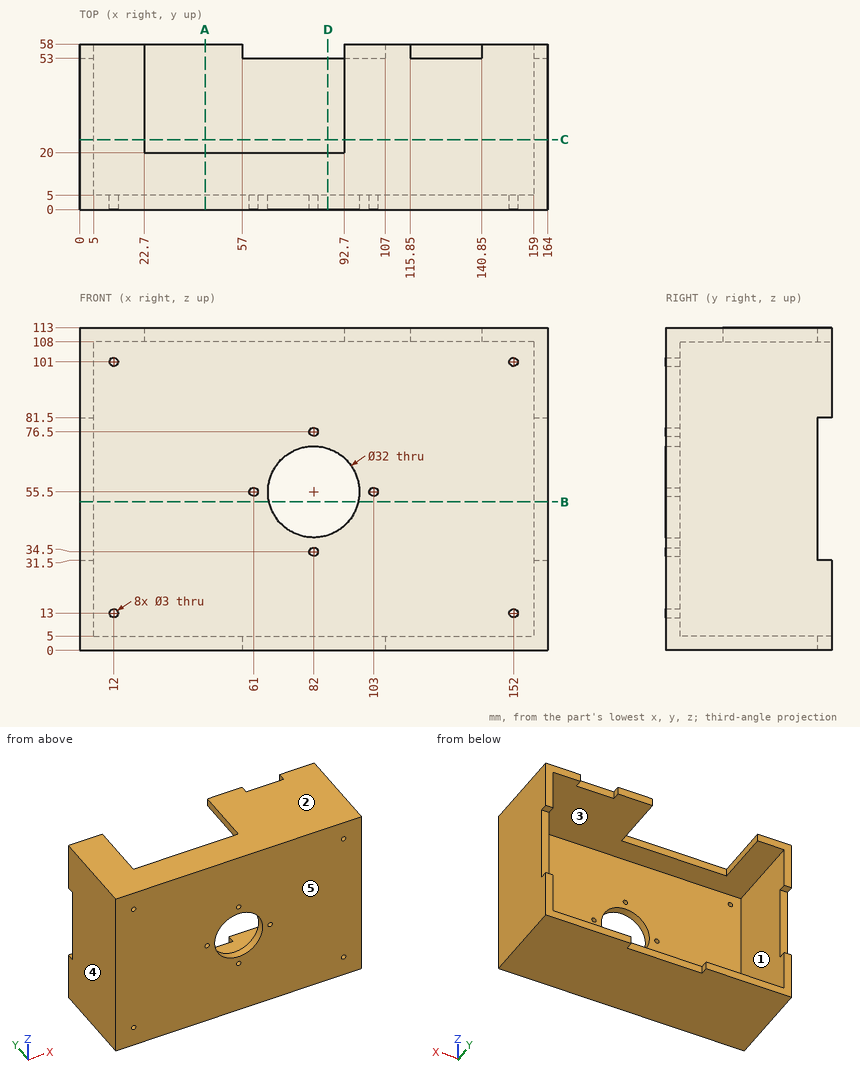
Drawing for the job (mm, zero at the part's lowest x, y, z). A direction names the side the tool comes from. Round coordinates to 2 decimals unless told otherwise and drop trailing zeros. Loops run counter-clockwise (first coordinate to the right, second up) from the corner with the lowest first, then second, coordinate; pieces in that order, holes last. Notation, with made-up numbers: (83, -1) -> (126, -1) arc R18 ccw to (126, 8) -> close; hole circle Ø2 at (-1.75, 38). An arc over 180 degrees is marked (long way). Answer in a Markdown table with one row per item.
Item 1: Saw through at D-D (x = 87). Write the cut outline in (y, z).
Answers below:
| item | result |
|---|---|
| outline | (0, 0) -> (53, 0) -> (53, 5) -> (5, 5) -> (5, 40.3) -> (0, 40.3) -> close; (0, 70.7) -> (5, 70.7) -> (5, 108) -> (20, 108) -> (20, 113) -> (0, 113) -> close |
Item 2: Saw through at C-C (y = 24.5). Write the cut outline in (x, z), and give its area (3 significant figures).
Answers below:
| item | result |
|---|---|
| outline | (0, 0) -> (164, 0) -> (164, 113) -> (92.7, 113) -> (92.7, 108) -> (159, 108) -> (159, 5) -> (5, 5) -> (5, 108) -> (22.7, 108) -> (22.7, 113) -> (0, 113) -> close |
| area | 2,320 mm² |
Item 3: Drill centre lines: L1, parallel to X at y = 3, z = 101; L2, parallel to Z at x = 152, y = 2; L3, parallel to X at y = 54, z = 13. Where is each one in solid material? Low to high. Write a range as [from, to].
Answers below:
| item | result |
|---|---|
| L1 | x = [0, 10.5], [13.5, 150.5], [153.5, 164] |
| L2 | z = [0, 11.5], [14.5, 99.5], [102.5, 113] |
| L3 | x = [0, 5], [159, 164] |
Item 4: Mould opens along X. For the marked faces 3, 4 and 5 say: +X half, -X half, draft (parallel to the pull), parting line (faces both ways), or undercut.
Answers below:
| item | result |
|---|---|
| face 3 | undercut |
| face 4 | -X half |
| face 5 | draft |
Item 5: Saw through at B-B (z = 52). Write the cut outline in (x, y), and give its area (3 significant figures).
Answers below:
| item | result |
|---|---|
| outline | (0, 0) -> (66.39, 0) -> (66.39, 5) -> (5, 5) -> (5, 53) -> (0, 53) -> close; (97.61, 0) -> (164, 0) -> (164, 53) -> (159, 53) -> (159, 5) -> (97.61, 5) -> close |
| area | 1,140 mm² |
Item 6: Which spindle directions (+Z, -Z, +X, -X, +Y, -Y) get a long thin tool onto all of the face, cutting with end or side? Do the marked faces 1 and 2. Say none if no direction does.
Answers below:
| item | result |
|---|---|
| face 1 | +Y |
| face 2 | +Z, +X, -X, +Y, -Y |
Item 7: Pin check, flat tips, straight feed: pin 1 (5.5 mm diameter, centred on x = 69.5, z = 111, fed in from +Y); pin 2 (3.5 mm diameter, centred on x = 103, z = 55.5, fed in from +Y). Stop position of each tip, or through.
Answers below:
| item | result |
|---|---|
| pin 1 | stops at y = 20 |
| pin 2 | stops at y = 5 |
Item 8: Saw through at A-A (x = 44). Write the cut outline in (y, z).
Answers below:
| item | result |
|---|---|
| outline | (0, 0) -> (58, 0) -> (58, 5) -> (5, 5) -> (5, 108) -> (20, 108) -> (20, 113) -> (0, 113) -> close |
